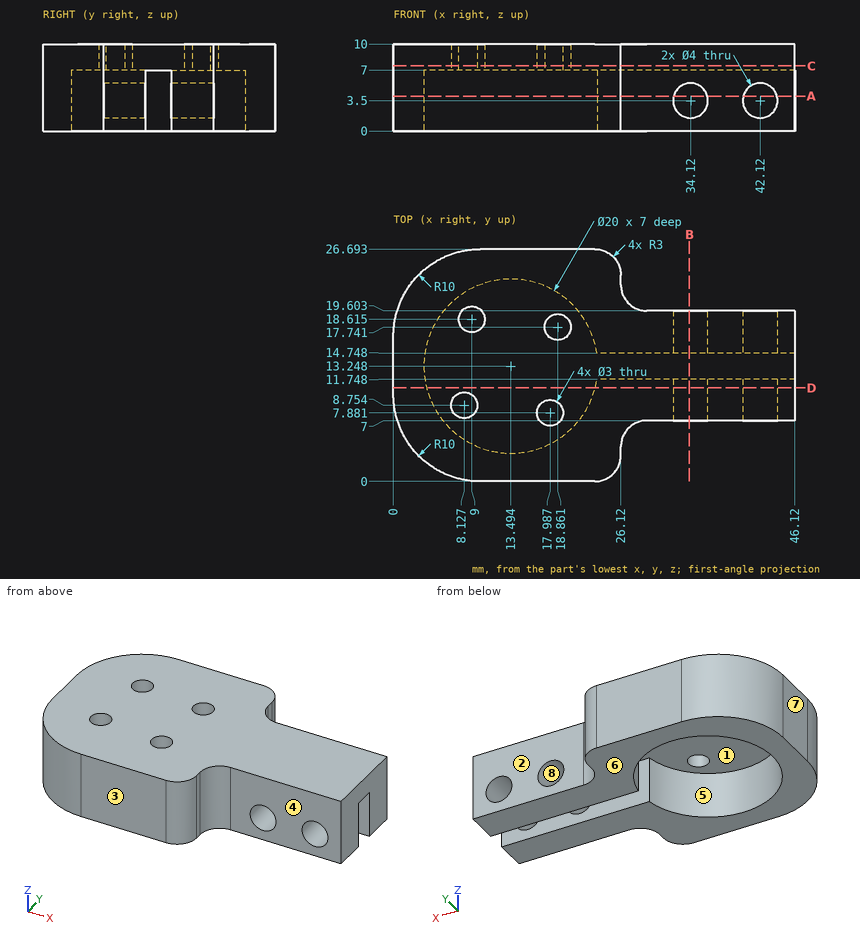
Verification items for this drawing (mm, ordinates from the low corner). A direction names the side the tool comes from. Give positions to 0.01 mm unless a question says otherwise; leave off trailing zeros. Write each loop counter-clockwise with the first axis right and the second up, starting at its lowest first coordinate (ties: lowest second). Pieces come first, ordered by that corner, then holes.
1) Thickness scan on line 1 (Z direction, x = 15.5, y = 14.5); line 2 (Y direction, x = 42.5, z = 1.25); line 3 (Y direction, x = 5.5, z = 4.25) (1 decimal). Record the ranges inside material, lowest first.
Values follow:
line 1: z = 7 to 10
line 2: y = 7 to 11.75, 14.75 to 19.6
line 3: y = 1.1 to 7.2, 19.3 to 25.6
2) Release check for a two-part mould opening along X. For the marked faces 5, 6, 7 and 8 record: released by +X, released by -X, zero draft, split by the parting line, or undercut.
Values follow:
face 5: undercut
face 6: zero draft
face 7: released by -X
face 8: undercut
3) Cross-section at A-A (z = 4). Count the separate pieces of the cut face and the enclosed holes in it, plus the area to 3 significant figures.
Values follow:
separate pieces: 5
enclosed holes: 0
area: 450 mm2
4) Cross-section at B-B (x = 34). Record the boundary of the cut face in (y, z).
Values follow:
outline: (7, 0) - (11.75, 0) - (11.75, 1.5) - (7, 1.5) - close; (7, 5.5) - (11.75, 5.5) - (11.75, 7) - (14.75, 7) - (14.75, 5.5) - (19.6, 5.5) - (19.6, 10) - (7, 10) - close; (14.75, 0) - (19.6, 0) - (19.6, 1.5) - (14.75, 1.5) - close
5) Cross-section at D-D (y = 10.75). Record the boundary of the cut face in (x, z).
Values follow:
outline: (0, 0) - (3.81, 0) - (3.81, 7) - (23.18, 7) - (23.18, 0) - (46.12, 0) - (46.12, 10) - (0, 10) - close; hole circle Ø4 at (34.12, 3.5); hole circle Ø4 at (42.12, 3.5)
6) Set-up check for the marked faces 1, 2, 3 and 4: record each of +Z, -Z, +X, -X, +Y, -Y from which the full face is reachable in a straight line by a thin tool's end or side.
Values follow:
face 1: -Z
face 2: +Z, -Z, +X, +Y
face 3: +Z, -Z, +X, -X, -Y
face 4: +Z, -Z, +X, -Y
7) Go/stop test with flat-tipped pins: pin 1 Ø0.9 at (y, z) = (23, 6.5) entering from +X; pin 2 Ø3.5 at (x, z) = (36.5, 2) entering from -Y; pin 3 Ø4 at (x, y) = (8.13, 8.75) entering from -Z; pin 4 Ø3.5 at (x, z) = (42.12, 3.5) entering from -Y (3 decimals). Record where each tip stops, or that it passes through.
Values follow:
pin 1: stops at x = 26.12
pin 2: stops at y = 7
pin 3: stops at z = 7
pin 4: passes through
8) Cross-section at C-C (z = 7.5). Record the boundary of the cut face in (x, y) (1 decimal).
Values follow:
outline: (0, 10) arc R10 ccw to (10, 0) - (23.1, 0) arc R3 ccw to (26.1, 3) - (26.1, 4) arc R3 cw to (29.1, 7) - (46.1, 7) - (46.1, 19.6) - (29.1, 19.6) arc R3 cw to (26.1, 22.6) - (26.1, 23.7) arc R3 ccw to (23.1, 26.7) - (10, 26.7) arc R10 ccw to (0, 16.7) - close; hole circle Ø3 at (8.1, 8.8); hole circle Ø3 at (9, 18.6); hole circle Ø3 at (18, 7.9); hole circle Ø3 at (18.9, 17.7)
